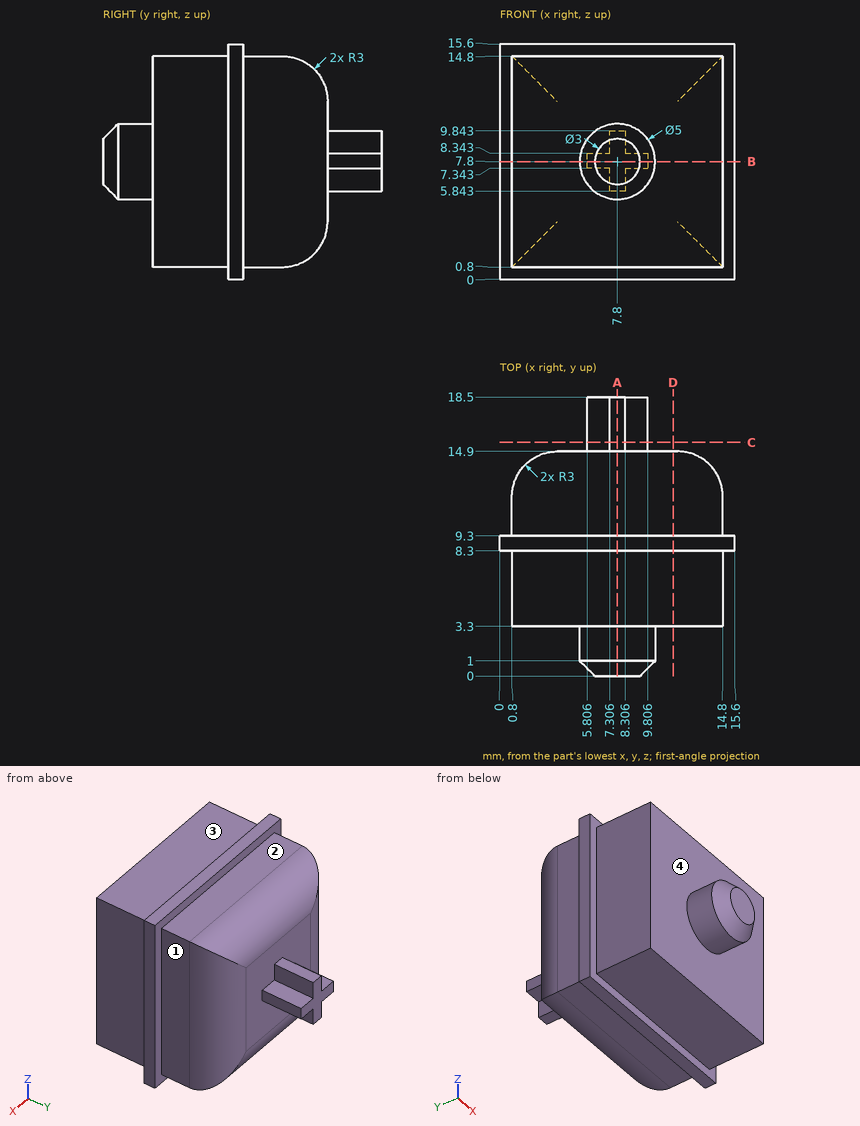
The drawing under review shows one solid part. Ordinate dimensions are in mm from its lowest x, y, z. A direction names the side the tool comes from. Give positions to 0.01 mm unless a question says otherwise; leave off trailing zeros. Write each loop counter-clockwise with the first axis right and the second up, starting at its lowest first coordinate (ties: lowest second). Pieces come first, ordered by that corner, then holes.
1. Add section D-D, the plane x = 11.5. Write out the cut boundary in (y, z).
2. Tool access review of the marked faces 1, 2, 3 and 4: name each direction out of +Z, -Z, +X, -X, +Y, -Y from which nothing blocks a thin tool from reaching the whole face with its end or side.
3. Add section A-A, the plane x = 7.8. Write out the cut boundary in (y, z).
4. Add section C-C, the plane y = 15.5. Write out the cut boundary in (x, z).
5. For P1, Ø5.5, axis at x = 9, y = 6, coming from the -Z side; P2, Ø1, axis at x = 12.5, y = 4, coming from the +Z side; P3, Ø1.6, axis at x = 9.5, y = 16, coming from the -Z side; P4, Ø1.5, axis at y = 6, z = 5, coming from the +X side, all flat-tipped, find the tip position at first contact; note any pin that passes through.
6. Add section B-B, the plane z = 7.8. Write out the cut boundary in (x, y), plus the area to 3 significant figures.
7. Wall thickness on L1, parallel to Y at x = 10, z = 4.5; L2, parallel to Z at x = 8.5, y = 11.25: over which ranges is each line inside the solid? List them lowest first.
Worked answers:
1. outline: (3.3, 0.8) - (8.3, 0.8) - (8.3, 0) - (9.3, 0) - (9.3, 0.8) - (11.9, 0.8) arc R3 ccw to (14.9, 3.8) - (14.9, 11.8) arc R3 ccw to (11.9, 14.8) - (9.3, 14.8) - (9.3, 15.6) - (8.3, 15.6) - (8.3, 14.8) - (3.3, 14.8) - close
2. face 1: +Z, -Z, +X, +Y
2. face 2: +Z, +X, -X, +Y
2. face 3: +Z, +X, -X, -Y
2. face 4: -Y
3. outline: (0, 6.3) - (1, 5.3) - (3.3, 5.3) - (3.3, 0.8) - (8.3, 0.8) - (8.3, 0) - (9.3, 0) - (9.3, 0.8) - (11.9, 0.8) arc R3 ccw to (14.9, 3.8) - (14.9, 5.84) - (18.5, 5.84) - (18.5, 9.84) - (14.9, 9.84) - (14.9, 11.8) arc R3 ccw to (11.9, 14.8) - (9.3, 14.8) - (9.3, 15.6) - (8.3, 15.6) - (8.3, 14.8) - (3.3, 14.8) - (3.3, 10.3) - (1, 10.3) - (0, 9.3) - close
4. outline: (5.81, 7.34) - (7.31, 7.34) - (7.31, 5.84) - (8.31, 5.84) - (8.31, 7.34) - (9.81, 7.34) - (9.81, 8.34) - (8.31, 8.34) - (8.31, 9.84) - (7.31, 9.84) - (7.31, 8.34) - (5.81, 8.34) - close
5. P1: stops at z = 0
5. P2: stops at z = 14.8
5. P3: stops at z = 7.34
5. P4: stops at x = 14.8
6. outline: (0, 8.3) - (0.8, 8.3) - (0.8, 3.3) - (5.3, 3.3) - (5.3, 1) - (6.3, 0) - (9.3, 0) - (10.3, 1) - (10.3, 3.3) - (14.8, 3.3) - (14.8, 8.3) - (15.6, 8.3) - (15.6, 9.3) - (14.8, 9.3) - (14.8, 11.9) arc R3 ccw to (11.8, 14.9) - (9.81, 14.9) - (9.81, 18.5) - (5.81, 18.5) - (5.81, 14.9) - (3.8, 14.9) arc R3 ccw to (0.8, 11.9) - (0.8, 9.3) - (0, 9.3) - close
6. area: 190 mm2
7. L1: y = 3.3 to 14.9
7. L2: z = 0.8 to 14.8
